Check sheet for the drawn part. Datum: minimum x, y, z corner. Units: mm. A direction names the side the tool comes from. Give positions to 0.01 mm unless a question says otherwise; leave off trailing zeros. Write each loop counter-clockwise with the first axis right and the second up, starting at its lowest first coordinate (ties: lowest second). Pieces come first, ordered by that corner, then holes. Notation, with made-up numbers: M 58,20 L 67,20 A16 cw 67,26 Z; hole C -30,22 d7. An arc over 180 degrees is marked long. Write item = value, one per line. Start each with the question number.
1) Sectioned sample at C-C, the plane y = 4. Count the separate pieces of the cut face and the enclosed holes in it, then the cut area to 3 significant figures.
2) Scan lines: L1, parallel to X at y = 4.25, z = 23; L2, parallel to Y at x = 16.5, z = 15; L3, parallel to Z at x = 21.5, y = 1.75. Record each from-to range of solid material in increasing order.
3) Sectioned sample at A-A, the plane x = 23. Record the cut outline in (y, z).
4) Set-up check for the marked faces 1 and 2: record each of +Z, -Z, +X, -X, +Y, -Y from which the full face is reachable in a straight line by a thin tool's end or side.
5) Sectioned sample at B-B, the plane z = 23. Record the cut outline in (x, y).
6) Gauge pin test, flat ends, axial feed: pin 1 (3 mm diameter, centred on x = 16.28, z = 29.72, fed in from -Y); pin 2 (3 mm diameter, centred on x = 8, y = 5, fed in from +Z); pin 3 (13 mm diameter, centred on x = 23, z = 23, fed in from -Y); pin 4 (1.5 mm diameter, centred on y = 4.5, z = 37, fed in from +X). Record the tip position at first contact, or that the pin passes through.
7) Sectioned sample at D-D, the plane x = 30. Record the cut outline in (y, z) (1 decimal).
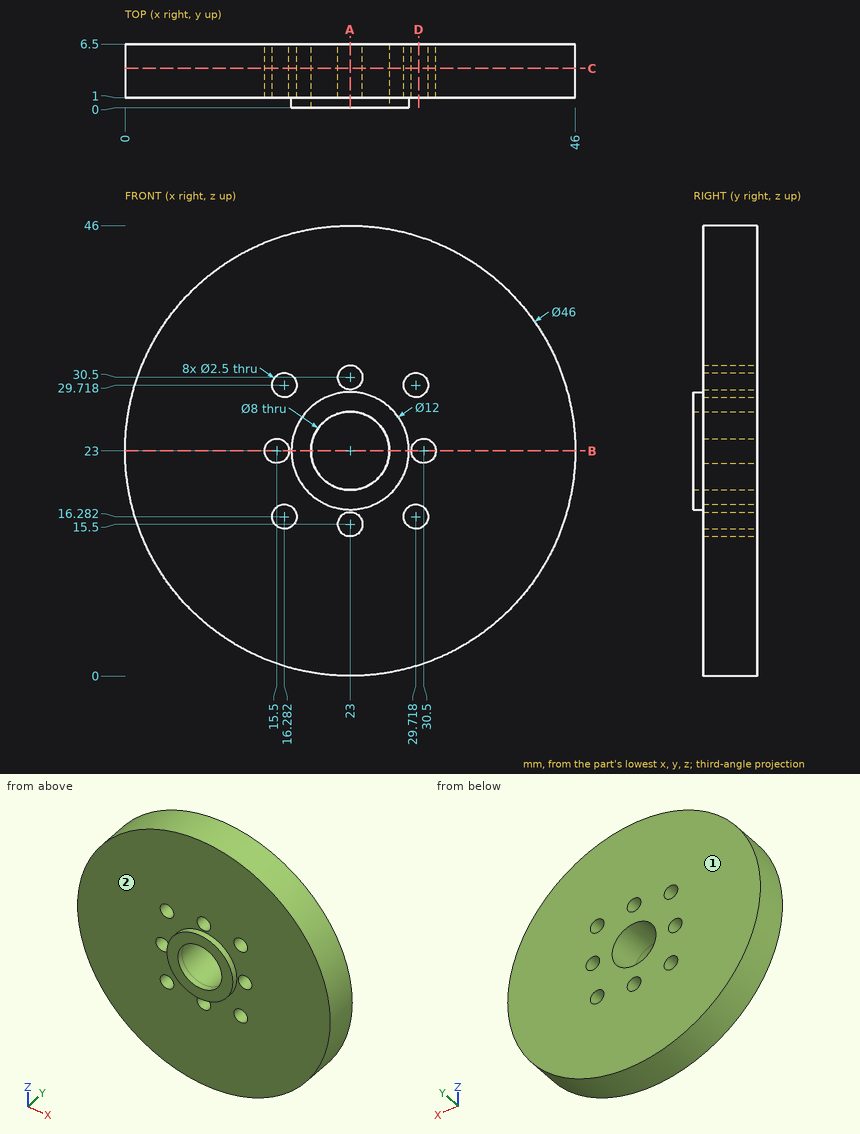
Data:
q1.separate_pieces = 1
q1.enclosed_holes = 9
q1.area = 1,570 mm2
q2.L1 = 0 to 14.25, 16.75 to 19, 27 to 29.25, 31.75 to 46
q2.L2 = 1 to 6.5
q2.L3 = 0.05 to 19.29, 26.71 to 45.95
q3.outline = M 0,17 L 1,17 L 1,16.75 L 6.5,16.75 L 6.5,19 L 0,19 Z; M 0,27 L 6.5,27 L 6.5,29.25 L 1,29.25 L 1,29 L 0,29 Z; M 1,0 L 6.5,0 L 6.5,14.25 L 1,14.25 Z; M 1,31.75 L 6.5,31.75 L 6.5,46 L 1,46 Z
q4.face_1 = +Z, -Z, +X, -X, +Y
q4.face_2 = -Y
q5.outline = M 0,1 L 14.25,1 L 14.25,6.5 L 0,6.5 Z; M 16.75,1 L 17,1 L 17,0 L 19,0 L 19,6.5 L 16.75,6.5 Z; M 27,0 L 29,0 L 29,1 L 29.25,1 L 29.25,6.5 L 27,6.5 Z; M 31.75,1 L 46,1 L 46,6.5 L 31.75,6.5 Z
q6.pin_1 = 1
q6.pin_2 = 41.62
q6.pin_3 = 0
q6.pin_4 = 41.8
q7.outline = M 1,1.1 L 6.5,1.1 L 6.5,15.1 L 1,15.1 Z; M 1,17.5 L 6.5,17.5 L 6.5,21.9 L 1,21.9 Z; M 1,24.1 L 6.5,24.1 L 6.5,28.5 L 1,28.5 Z; M 1,30.9 L 6.5,30.9 L 6.5,44.9 L 1,44.9 Z
